Design review of the part built by this model. Coordinates are the model's own, in mm. A direction names the side the tool comes from. Give positions to 0.01 mm unless a question says otherwise; leave off trailing zeros. Loops run counter-clockwise (first coordinate to the right, second up) from the corner with the lowest first, then second, coordinate; pieces in that order, holes last. Notation, with made-up numbers: (-37.75, -27) - (12.25, -27) arc R20 cw to (12.25, 7) - close; hole circle Ø9 at (-16, 0). An arc over 180 degrees is marked (long way). Write each question's results on one line, items separated by ' | '.
```python
from build123d import *

# Parameters (mm, degrees)
SKETCH1_R                 = 1.143
BOSS_EXTRUDE1_DEPTH       = 3.9624
SKETCH2_W                 = 6.35
SKETCH2_H                 = 4.7752
BOSS_EXTRUDE2_DEPTH       = 3.4036
BOSS_EXTRUDE3_DEPTH       = 0.127
BOSS_EXTRUDE3_DEPTH_BACK  = 0.127
SKETCH3_R                 = 0.5588
BOSS_EXTRUDE4_DEPTH       = 0.127
BOSS_EXTRUDE4_DEPTH_BACK  = 0.127
SKETCH4_R                 = 0.5588
BOSS_EXTRUDE5_DEPTH       = 0.127
BOSS_EXTRUDE5_DEPTH_BACK  = 0.127
SKETCH5_R                 = 0.5588
BOSS_EXTRUDE6_DEPTH       = 0.127
BOSS_EXTRUDE6_DEPTH_BACK  = 0.127
SKETCH7_R                 = 0.5588
BOSS_EXTRUDE7_DEPTH       = 0.127
BOSS_EXTRUDE7_DEPTH_BACK  = 0.127
SKETCH6_R                 = 0.5588
BOSS_EXTRUDE8_DEPTH       = 0.0508
BOSS_EXTRUDE8_DEPTH_BACK  = 0.0508
BOSS_EXTRUDE11_DEPTH      = 0.0508
BOSS_EXTRUDE11_DEPTH_BACK = 0.0508
BOSS_EXTRUDE12_DEPTH      = 0.0508
BOSS_EXTRUDE12_DEPTH_BACK = 0.0508
BOSS_EXTRUDE13_DEPTH      = 0.0508
BOSS_EXTRUDE13_DEPTH_BACK = 0.0508
BOSS_EXTRUDE14_DEPTH      = 0.0508
BOSS_EXTRUDE14_DEPTH_BACK = 0.0508


with BuildPart() as part:
    # Sketch1 → Boss-Extrude1 (new body)
    with BuildSketch(Plane.XY):
        with BuildLine():
            Line((-5.5499, 2.3876), (5.5499, 2.3876))
            ThreePointArc((5.5499, 2.3876), (7.9375, 0), (5.5499, -2.3876))
            Line((5.5499, -2.3876), (-5.5499, -2.3876))
            ThreePointArc((-5.5499, -2.3876), (-7.9375, 0), (-5.5499, 2.3876))
        make_face()
        with Locations((-5.5499, 0)):
            Circle(SKETCH1_R, mode=Mode.SUBTRACT)
        with Locations((5.5499, 0)):
            Circle(SKETCH1_R, mode=Mode.SUBTRACT)
    extrude(amount=BOSS_EXTRUDE1_DEPTH)

    # Sketch2 → Boss-Extrude2 (add)
    with BuildSketch(Plane.XY.offset(3.9624)):
        Rectangle(SKETCH2_W, SKETCH2_H)
    extrude(amount=BOSS_EXTRUDE2_DEPTH)

    # Sketch3 → Boss-Extrude3 (add, two sides: drawn at the far end of the back side and taken through both)
    with BuildSketch(Plane(origin=(0, 0, 1.651), x_dir=(-1, 0, 0), z_dir=(0, 0, -1)).offset(-BOSS_EXTRUDE3_DEPTH_BACK)):
        with BuildLine():
            Line((-2.3114, 3.5941), (-2.3114, 2.3876))
            Line((-2.3114, 2.3876), (0, 2.3876))
            Line((0, 2.3876), (0, 3.5941))
            ThreePointArc((0, 3.5941), (-1.1557, 4.7498), (-2.3114, 3.5941))
        make_face()
        with Locations((-1.1557, 3.5941)):
            Circle(SKETCH3_R, mode=Mode.SUBTRACT)
    extrude(amount=BOSS_EXTRUDE3_DEPTH + BOSS_EXTRUDE3_DEPTH_BACK)

    # Sketch4 → Boss-Extrude4 (add, two sides: drawn at the far end of the back side and taken through both)
    with BuildSketch(Plane(origin=(0, 0, 2.921), x_dir=(-1, 0, 0), z_dir=(0, 0, -1)).offset(-BOSS_EXTRUDE4_DEPTH_BACK)):
        with BuildLine():
            Line((2.3114, 3.5941), (2.3114, 2.3876))
            Line((2.3114, 2.3876), (0, 2.3876))
            Line((0, 2.3876), (0, 3.5941))
            ThreePointArc((0, 3.5941), (1.1557, 4.7498), (2.3114, 3.5941))
        make_face()
        with Locations(Location((1.1557, 3.5941, 0), (0, 0, 180))):
            Circle(SKETCH4_R, mode=Mode.SUBTRACT)
    extrude(amount=BOSS_EXTRUDE4_DEPTH + BOSS_EXTRUDE4_DEPTH_BACK)

    # Sketch5 → Boss-Extrude5 (add, two sides: drawn at the far end of the back side and taken through both)
    with BuildSketch(Plane(origin=(0, 0, 4.191), x_dir=(-1, 0, 0), z_dir=(0, 0, -1)).offset(-BOSS_EXTRUDE5_DEPTH_BACK)):
        with BuildLine():
            Line((-2.3114, 3.5941), (-2.3114, 2.3876))
            Line((-2.3114, 2.3876), (0, 2.3876))
            Line((0, 2.3876), (0, 3.5941))
            ThreePointArc((0, 3.5941), (-1.1557, 4.7498), (-2.3114, 3.5941))
        make_face()
        with Locations((-1.1557, 3.5941)):
            Circle(SKETCH5_R, mode=Mode.SUBTRACT)
    extrude(amount=BOSS_EXTRUDE5_DEPTH + BOSS_EXTRUDE5_DEPTH_BACK)

    # Sketch7 → Boss-Extrude6 (add, two sides: drawn at the far end of the back side and taken through both)
    with BuildSketch(Plane(origin=(0, 0, 5.461), x_dir=(-1, 0, 0), z_dir=(0, 0, -1)).offset(-BOSS_EXTRUDE6_DEPTH_BACK)):
        with BuildLine():
            Line((2.3114, 2.3876), (2.3114, 3.5941))
            ThreePointArc((2.3114, 3.5941), (1.1557, 4.7498), (0, 3.5941))
            Line((0, 3.5941), (0, 2.3876))
            Line((0, 2.3876), (2.3114, 2.3876))
        make_face()
        with Locations(Location((1.1557, 3.5941, 0), (0, 0, 180))):
            Circle(SKETCH7_R, mode=Mode.SUBTRACT)
    extrude(amount=BOSS_EXTRUDE6_DEPTH + BOSS_EXTRUDE6_DEPTH_BACK)

    # Sketch6 → Boss-Extrude7 (add, two sides: drawn at the far end of the back side and taken through both)
    with BuildSketch(Plane(origin=(0, 0, 6.731), x_dir=(-1, 0, 0), z_dir=(0, 0, -1)).offset(-BOSS_EXTRUDE7_DEPTH_BACK)):
        with BuildLine():
            Line((-2.3114, 3.5941), (-2.3114, 2.3876))
            Line((-2.3114, 2.3876), (0, 2.3876))
            Line((0, 2.3876), (0, 3.5941))
            ThreePointArc((0, 3.5941), (-1.1557, 4.7498), (-2.3114, 3.5941))
        make_face()
        with Locations((-1.1557, 3.5941)):
            Circle(SKETCH6_R, mode=Mode.SUBTRACT)
    extrude(amount=BOSS_EXTRUDE7_DEPTH + BOSS_EXTRUDE7_DEPTH_BACK)

    # Sketch8 → Boss-Extrude8 (add, two sides: drawn at the far end of the back side and taken through both)
    with BuildSketch(Plane(origin=(0, 0, 1.651), x_dir=(-1, 0, 0), z_dir=(0, 0, -1)).offset(-BOSS_EXTRUDE8_DEPTH_BACK)):
        Polygon((2.228681211, -2.3876), (2.028101851, -2.3876), (0.796265448, -10.3124), (0.900870757, -10.3124), align=None)
        Polygon((-0.900870757, -10.3124), (-0.796265448, -10.3124), (-2.028101851, -2.3876), (-2.228681211, -2.3876), align=None)
    extrude(amount=BOSS_EXTRUDE8_DEPTH + BOSS_EXTRUDE8_DEPTH_BACK)

    # Sketch11 → Boss-Extrude11 (add, two sides: drawn at the far end of the back side and taken through both)
    with BuildSketch(Plane(origin=(0, 0, 4.191), x_dir=(-1, 0, 0), z_dir=(0, 0, -1)).offset(-BOSS_EXTRUDE11_DEPTH_BACK)):
        Polygon((2.228681211, -2.3876), (0.900870757, -10.3124), (0.796265448, -10.3124), (2.028101851, -2.3876), align=None)
        Polygon((-0.900870757, -10.3124), (-0.796265448, -10.3124), (-2.028101851, -2.3876), (-2.228681211, -2.3876), align=None)
    extrude(amount=BOSS_EXTRUDE11_DEPTH + BOSS_EXTRUDE11_DEPTH_BACK)

    # Sketch12 → Boss-Extrude12 (add, two sides: drawn at the far end of the back side and taken through both)
    with BuildSketch(Plane(origin=(0, 0, 6.731), x_dir=(-1, 0, 0), z_dir=(0, 0, -1)).offset(-BOSS_EXTRUDE12_DEPTH_BACK)):
        Polygon((2.228681211, -2.3876), (0.900870757, -10.3124), (0.796265448, -10.3124), (2.028101851, -2.3876), align=None)
        Polygon((-0.900870757, -10.3124), (-0.796265448, -10.3124), (-2.028101851, -2.3876), (-2.228681211, -2.3876), align=None)
    extrude(amount=BOSS_EXTRUDE12_DEPTH + BOSS_EXTRUDE12_DEPTH_BACK)

    # Sketch13 → Boss-Extrude13 (add, two sides: drawn at the far end of the back side and taken through both)
    with BuildSketch(Plane(origin=(0, 0, 2.921), x_dir=(-1, 0, 0), z_dir=(0, 0, -1)).offset(-BOSS_EXTRUDE13_DEPTH_BACK)):
        Polygon((0.900870757, -10.3124), (0.796265448, -10.3124), (2.028101851, -2.3876), (2.228681211, -2.3876), align=None)
        Polygon((-0.900870757, -10.3124), (-0.796265448, -10.3124), (-2.028101851, -2.3876), (-2.228681211, -2.3876), align=None)
    extrude(amount=BOSS_EXTRUDE13_DEPTH + BOSS_EXTRUDE13_DEPTH_BACK)

    # Sketch15 → Boss-Extrude14 (add, two sides: drawn at the far end of the back side and taken through both)
    with BuildSketch(Plane(origin=(0, 0, 5.461), x_dir=(-1, 0, 0), z_dir=(0, 0, -1)).offset(-BOSS_EXTRUDE14_DEPTH_BACK)):
        Polygon((-0.900870757, -10.3124), (-2.228681211, -2.3876), (-2.028101851, -2.3876), (-0.796265448, -10.3124), align=None)
        Polygon((0.796265448, -10.3124), (0.900870757, -10.3124), (2.228681211, -2.3876), (2.028101851, -2.3876), align=None)
    extrude(amount=BOSS_EXTRUDE14_DEPTH + BOSS_EXTRUDE14_DEPTH_BACK)


solid = part.part
```
Item 1: Wall thickness on probe 1 along Y at (x, z) = (-2, 1.75); probe 2 along Z at (x, y) = (-1.25, 3); probe 3 along Z at (x, y) = (5, 1.75): over which ranges is each line inside the solid? List them lowest first.
Output values:
probe 1: y = -2.39 to 2.39 | probe 2: z = 2.79 to 3.05, 5.33 to 5.59 | probe 3: z = 0 to 3.96
Item 2: We need section D-D on y = 1.75. Give the boundary of the cut face in (x, z) (3 decimals), then the cut area to 3 significant figures.
Output values:
outline: (-7.174, 0) - (7.174, 0) - (7.174, 3.962) - (3.175, 3.962) - (3.175, 7.366) - (-3.175, 7.366) - (-3.175, 3.962) - (-7.174, 3.962) - close | area: 78.5 mm²
Item 3: We need section C-C on x = 6.25. Give the boundary of the cut face in (y, z).
Output values:
outline: (-2.28, 0) - (-0.9, 0) - (-0.9, 3.96) - (-2.28, 3.96) - close; (0.9, 0) - (2.28, 0) - (2.28, 3.96) - (0.9, 3.96) - close
Item 4: Draft analysis for pull direction Z (two halves, no side actions). For faces 1 (the face through (-2, 3, 2.794)), 2 (the face through (2, 3, 1.778)), 3 (the face through (-7.937, -0.053, 1.953)), state which applies: +Z half, -Z half, draft (parallel to the pull), parting line (faces both ways), or undercut.
Output values:
face 1: -Z half | face 2: undercut | face 3: draft
Item 5: Clearance check with flat-ended pins moving along their axes: P1, Ø0.7, axis at x = 2, y = -5, coming from the +Z side; P2, Ø0.7, axis at x = 1.5, y = -6, coming from the -Z side; P3, Ø1.1, axis at x = -1, y = -5, coming from the +Z side; P4, Ø1.5, axis at y = 2.5, z = 1, coming from the +X side. State where each tip first meets the part, or that it passes through.
Output values:
P1: stops at z = 6.78 | P2: stops at z = 1.6 | P3: passes through | P4: stops at x = 7.17
Item 6: Tool access review of faces 4 (the face through (2, 3, 4.064)), 5 (the face through (3.175, 0, 6)): name each direction out of +Z, -Z, +X, -X, +Y, -Y from which nothing blocks a thin tool from reaching the whole face with its end or side.
Output values:
face 4: +X, -X, +Y | face 5: +Z, +X, +Y, -Y
Item 7: We need section A-A on y = 0. Give the boundary of the cut face in (x, z) (1 decimal), then the cut area to 3 significant figures.
Output values:
outline: (-7.9, 0) - (-6.7, 0) - (-6.7, 4) - (-7.9, 4) - close; (-4.4, 0) - (4.4, 0) - (4.4, 4) - (3.2, 4) - (3.2, 7.4) - (-3.2, 7.4) - (-3.2, 4) - (-4.4, 4) - close; (6.7, 0) - (7.9, 0) - (7.9, 4) - (6.7, 4) - close | area: 66.4 mm²
Item 8: We need section B-B on z = 0.5. Give the boundary of the cut face in (x, y), then the cut area to 3 significant figures.
Output values:
outline: (-5.55, -2.39) - (5.55, -2.39) arc R2.39 ccw to (5.55, 2.39) - (-5.55, 2.39) arc R2.39 ccw to start; hole circle Ø2.29 at (-5.55, 0); hole circle Ø2.29 at (5.55, 0) | area: 62.7 mm²
